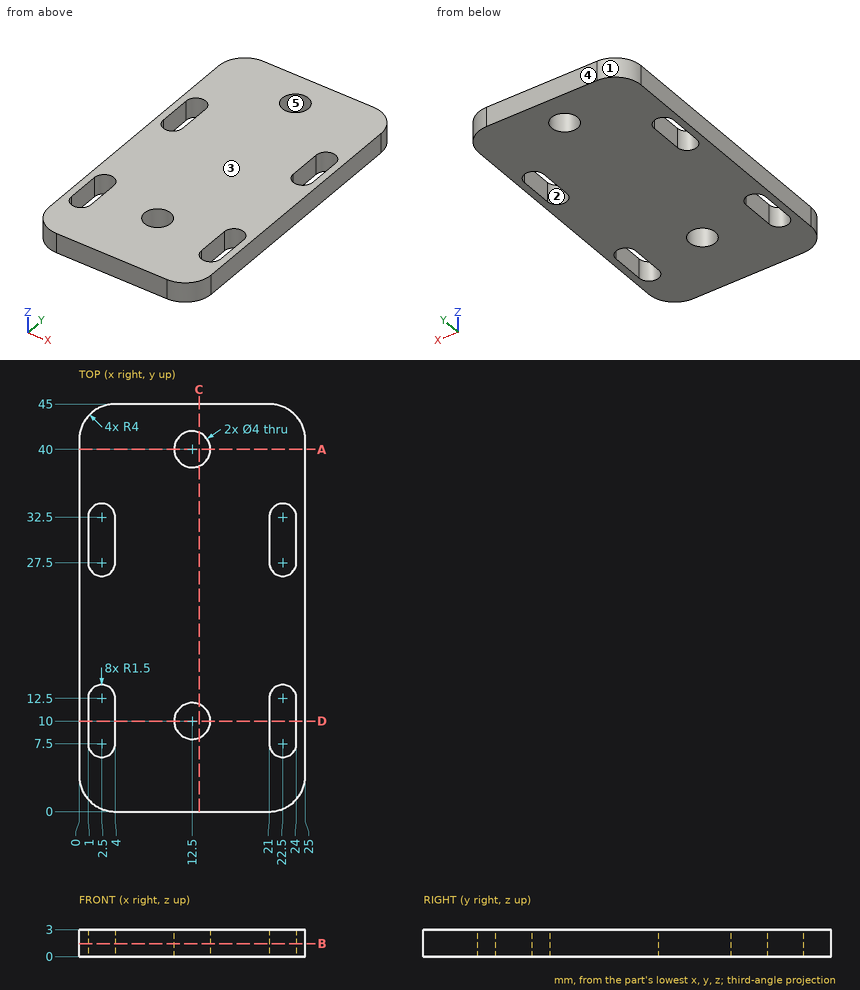
Geometry: see drawing. Coordinates: mm, zero at the bounding-box minimum. A direction names the side the tool comes from. Round coordinates to 2 decimals unless told otherwise and drop trailing zeros. Order: outer loops, then holes, each group sorted by start corner. A loop starts at its lowest first (then second) coordinate and runs counter-clockwise, first axis right, second up. Notation, with made-up numbers: (9, -16.75) - (56, -16.75) arc R8 cw to (56, -4.75) - close; hole circle Ø6 at (-15, 54.25). An arc over 180 degrees is marked (long way). One line per question, with ' | ' between items. Start each with the question number.
1) Cut plane A-A, the plane y = 40. Return the cut outline in (x, z).
2) Pull-direction query (Y, two-part tool) for the marked faces 3, 4 and 5; classes: +Y half, -Y half, draft (parallel to the pull), parting line (faces both ways), or undercut.
3) Cut plane C-C, the plane x = 13.25. Return the cut outline in (y, z).
4) Cut plane B-B, the plane z = 1.45. Return the cut outline in (x, y), then the cut area to 3 significant figures.
5) Set-up query: the marked faces 1 and 2. Return all of +Z, -Z, +X, -X, +Y, -Y with unobstructed straight access to the full face (end or side cutting, diameter ignored); none if empty.
6) Ray query, probe 1 along Y at (x, z) = (12.5, 1.25); probe 2 along X at (y, z) = (7.5, 0.4); probe 3 along Y at (x, z) = (21.5, 2.65). Return the intervals inside material, ascending.
7) Cut plane D-D, the plane y = 10. Return the cut outline in (x, z).
Worked out:
1) outline: (0, 0) - (10.5, 0) - (10.5, 3) - (0, 3) - close; (14.5, 0) - (25, 0) - (25, 3) - (14.5, 3) - close
2) face 3: draft | face 4: +Y half | face 5: undercut
3) outline: (0, 0) - (8.15, 0) - (8.15, 3) - (0, 3) - close; (11.85, 0) - (38.15, 0) - (38.15, 3) - (11.85, 3) - close; (41.85, 0) - (45, 0) - (45, 3) - (41.85, 3) - close
4) outline: (0, 4) arc R4 ccw to (4, 0) - (21, 0) arc R4 ccw to (25, 4) - (25, 41) arc R4 ccw to (21, 45) - (4, 45) arc R4 ccw to (0, 41) - close; hole (1, 7.5) arc R1.5 ccw to (4, 7.5) - (4, 12.5) arc R1.5 ccw to (1, 12.5) - close; hole (1, 27.5) arc R1.5 ccw to (4, 27.5) - (4, 32.5) arc R1.5 ccw to (1, 32.5) - close; hole circle Ø4 at (12.5, 10); hole circle Ø4 at (12.5, 40); hole (21, 7.5) arc R1.5 ccw to (24, 7.5) - (24, 12.5) arc R1.5 ccw to (21, 12.5) - close; hole (21, 27.5) arc R1.5 ccw to (24, 27.5) - (24, 32.5) arc R1.5 ccw to (21, 32.5) - close | area: 998 mm^2
5) face 1: +Z, -Z, -X, +Y | face 2: +Z, -Z
6) probe 1: y = 0 to 8, 12 to 38, 42 to 45 | probe 2: x = 0 to 1, 4 to 21, 24 to 25 | probe 3: y = 0.03 to 6.38, 13.62 to 26.38, 33.62 to 44.97
7) outline: (0, 0) - (1, 0) - (1, 3) - (0, 3) - close; (4, 0) - (10.5, 0) - (10.5, 3) - (4, 3) - close; (14.5, 0) - (21, 0) - (21, 3) - (14.5, 3) - close; (24, 0) - (25, 0) - (25, 3) - (24, 3) - close
